from build123d import *

# Parameters (mm, degrees)
SKETCH1_R           = 43
BOSS_EXTRUDE1_DEPTH = 3
BOSS_EXTRUDE2_DEPTH = 20
BOSS_EXTRUDE3_DEPTH = 3


with BuildPart() as part:
    # Sketch1 → Boss-Extrude1 (new body)
    with BuildSketch(Plane(origin=(0, 0, 0), x_dir=(1, 0, 0), z_dir=(0, 1, 0))):
        with Locations(Location((0, 0, 0), (0, 0, 270))):
            Circle(SKETCH1_R)
    extrude(amount=BOSS_EXTRUDE1_DEPTH)

    # Sketch2 → Boss-Extrude2 (add)
    with BuildSketch(Plane(origin=(0, 3, 0), x_dir=(1, 0, 0), z_dir=(0, 1, 0))):
        with BuildLine():
            Line((-43, 0), (-39.99995453, 0))
            ThreePointArc((-39.99995453, 0), (-39.961883436, 1.744773511), (-39.847742626, 3.486225747))
            Line((-39.847742626, 3.486225747), (-42.836372018, 3.747696938))
            ThreePointArc((-42.836372018, 3.747696938), (-42.959073528, 1.875633657), (-43, 0))
        make_face()
        with BuildLine():
            ThreePointArc((-39.847742626, -3.486225747), (-39.961883436, -1.744773511), (-39.99995453, 0))
            Line((-39.99995453, 0), (-43, 0))
            ThreePointArc((-43, 0), (-42.959073528, -1.875633657), (-42.836372018, -3.747696938))
            Line((-42.836372018, -3.747696938), (-39.847742626, -3.486225747))
        make_face()
        with BuildLine():
            ThreePointArc((39.847742626, 3.486225747), (39.961883436, 1.744773511), (39.99995453, 0))
            Line((39.99995453, 0), (43, 0))
            ThreePointArc((43, 0), (42.959073528, 1.875633657), (42.836372018, 3.747696938))
            Line((42.836372018, 3.747696938), (39.847742626, 3.486225747))
        make_face()
        with BuildLine():
            Line((43, 0), (39.99995453, 0))
            ThreePointArc((39.99995453, 0), (39.961883436, -1.744773511), (39.847742626, -3.486225747))
            Line((39.847742626, -3.486225747), (42.836372018, -3.747696938))
            ThreePointArc((42.836372018, -3.747696938), (42.959073528, -1.875633657), (43, 0))
        make_face()
        with BuildLine():
            Line((0, 43), (0, 39.99995453))
            ThreePointArc((0, 39.99995453), (1.744773511, 39.961883436), (3.486225747, 39.847742626))
            Line((3.486225747, 39.847742626), (3.747696938, 42.836372018))
            ThreePointArc((3.747696938, 42.836372018), (1.875633657, 42.959073528), (0, 43))
        make_face()
        with BuildLine():
            ThreePointArc((-3.486225747, 39.847742626), (-1.744773511, 39.961883436), (0, 39.99995453))
            Line((0, 39.99995453), (0, 43))
            ThreePointArc((0, 43), (-1.875633657, 42.959073528), (-3.747696938, 42.836372018))
            Line((-3.747696938, 42.836372018), (-3.486225747, 39.847742626))
        make_face()
    extrude(amount=BOSS_EXTRUDE2_DEPTH)

    # Sketch3 → Boss-Extrude3 (add)
    with BuildSketch(Plane(origin=(0, 23, 0), x_dir=(1, 0, 0), z_dir=(0, 1, 0))):
        with BuildLine():
            Line((-42.836372018, -3.747696938), (-39.847742626, -3.486225747))
            Line((-39.847742626, -3.486225747), (-24.755731256, -3.486225747))
            ThreePointArc((-24.755731256, -3.486225747), (0, -25), (24.755731256, -3.486225747))
            Line((24.755731256, -3.486225747), (39.847742626, -3.486225747))
            Line((39.847742626, -3.486225747), (42.836372018, -3.747696938))
            ThreePointArc((42.836372018, -3.747696938), (43, 0), (42.836372018, 3.747696938))
            Line((42.836372018, 3.747696938), (39.847742626, 3.486225747))
            Line((39.847742626, 3.486225747), (24.755731256, 3.486225747))
            ThreePointArc((24.755731256, 3.486225747), (17.67766953, 17.67766953), (3.486225747, 24.755731256))
            Line((3.486225747, 24.755731256), (3.486225747, 39.847742626))
            Line((3.486225747, 39.847742626), (3.747696938, 42.836372018))
            ThreePointArc((3.747696938, 42.836372018), (0, 43), (-3.747696938, 42.836372018))
            Line((-3.747696938, 42.836372018), (-3.486225747, 39.847742626))
            Line((-3.486225747, 39.847742626), (-3.486225747, 24.755731256))
            ThreePointArc((-3.486225747, 24.755731256), (-17.67766953, 17.67766953), (-24.755731256, 3.486225747))
            Line((-24.755731256, 3.486225747), (-39.847742626, 3.486225747))
            Line((-39.847742626, 3.486225747), (-42.836372018, 3.747696938))
            ThreePointArc((-42.836372018, 3.747696938), (-43, 0), (-42.836372018, -3.747696938))
        make_face()
    extrude(amount=BOSS_EXTRUDE3_DEPTH)


solid = part.part
Geometry check sheet. Reference: the model listing, model coordinates, mm. A direction names the side the tool comes from. Round coordinates to 2 decimals unless told otherwise and drop trailing zeros. Write each loop counter-clockwise with the first axis right and the second up, starting at its lowest first coordinate (ties: lowest second). Pieces come first, ordered by that corner, then holes.
Item 1: Go/stop test with flat-tipped pins: pin 1 Ø0.9 at (x, y) = (30.5, 24.5) entering from +Z; pin 2 Ø1.5 at (y, z) = (24.5, -36) entering from +X; pin 3 Ø3.5 at (y, z) = (25, -31.5) entering from -X. Record where each tip stops, or that it passes through.
Determined:
pin 1: stops at z = 3.49
pin 2: stops at x = 3.49
pin 3: stops at x = -3.49
Item 2: Material ranges on line 1 along Y through (x, z) = (2.5, -20); line 2 along Z through (x, y) = (-25, 23.25); line 3 along Y through (x, z) = (23.5, 22), recorded low to high.
Determined:
line 1: y = 0 to 3, 23 to 26
line 2: z = -3.49 to 3.49
line 3: y = 0 to 3
Item 3: Access from +Z, -Z, +X, -X, +Y, -Y to the whole of each face (thin tool, end or side, straight path). Record for faces 4 (the face through (-41.321, 14.339, -3.615)), 5 (the face through (41.321, 14.339, 3.615)), 6 (the face through (3.486, 24, -32)), 7 (the face through (-3.486, 24, -32)).
Determined:
face 4: -Z, +Y
face 5: +Z, +Y
face 6: +X, +Y
face 7: -X, +Y
Item 4: Section check D-D (z = 34.5). Record the boundary of the cut face in (x, y).
Determined:
outline: (-25.67, 0) - (25.67, 0) - (25.67, 3) - (-25.67, 3) - close
Item 5: Section check B-B (z = -31.5). Record the boundary of the cut face in (x, y).
Determined:
outline: (-29.27, 0) - (29.27, 0) - (29.27, 3) - (-29.27, 3) - close; (-3.49, 23) - (3.49, 23) - (3.49, 26) - (-3.49, 26) - close
Item 6: Mould release check, pull along Y, two halves, no side actions. Record for faces 1 (the face through (1, 3, -1)), 2 (the face through (1, 0, -1)), 3 (the face through (32, 24, 3.486)): +Y half, -Y half, draft (parallel to the pull), parting line (faces both ways), or undercut.
Determined:
face 1: undercut
face 2: -Y half
face 3: draft
Item 7: Section check C-C (x = 36). Record the boundary of the cut face in (y, z), plus the area to 3 significant figures.
Determined:
outline: (0, -23.52) - (3, -23.52) - (3, 23.52) - (0, 23.52) - close; (23, -3.49) - (26, -3.49) - (26, 3.49) - (23, 3.49) - close
area: 162 mm2
Item 8: Section check A-A (y = 8.5). Record the boundary of the cut face in (x, z), plus the area to 3 significant figures.
Determined:
outline: (-42.84, -3.75) - (-39.85, -3.49) arc R40 cw to (-39.85, 3.49) - (-42.84, 3.75) arc R43 ccw to start; (-3.75, -42.84) arc R43 ccw to (3.75, -42.84) - (3.49, -39.85) arc R40 cw to (-3.49, -39.85) - close; (39.85, -3.49) - (42.84, -3.75) arc R43 ccw to (42.84, 3.75) - (39.85, 3.49) arc R40 cw to start
area: 65.2 mm2
